from build123d import *

# Parameters (mm, degrees)
F0_R     = 3.5
F0_R_2   = 1.5
F1_DEPTH = 20
F2_W     = 5
F2_H     = 30
F3_DEPTH = 5


with BuildPart() as f1:
    # F0 (on Top) → F1 (new body)
    with BuildSketch(Plane.XY):
        Polygon((-10, 15), (-15, 15), (-15, -15), (-10, -15), (10, -15), (15, -15), (15, 15), (10, 15), align=None)
        with Locations((-5, -7.9105878249)):
            Circle(F0_R, mode=Mode.SUBTRACT)
        with Locations((5, -5.0300965086)):
            Circle(F0_R, mode=Mode.SUBTRACT)
        with Locations((-5, 0)):
            Circle(F0_R, mode=Mode.SUBTRACT)
        with Locations((-5, 7.8226719052)):
            Circle(F0_R, mode=Mode.SUBTRACT)
        with Locations((5, 4.2056075387)):
            Circle(F0_R, mode=Mode.SUBTRACT)
        with Locations((5, 4.2056075387)):
            Circle(F0_R)
        with Locations((5, 4.2056075387)):
            Circle(F0_R_2, mode=Mode.SUBTRACT)
        with Locations((-5, 7.8226719052)):
            Circle(F0_R)
        with Locations((-5, 7.8226719052)):
            Circle(F0_R_2, mode=Mode.SUBTRACT)
        with Locations((-5, 0)):
            Circle(F0_R)
        with Locations((-5, 0)):
            Circle(F0_R_2, mode=Mode.SUBTRACT)
        with Locations((-5, -7.9105878249)):
            Circle(F0_R)
        with Locations((-5, -7.9105878249)):
            Circle(F0_R_2, mode=Mode.SUBTRACT)
        with Locations((5, -5.0300965086)):
            Circle(F0_R)
        with Locations((5, -5.0300965086)):
            Circle(F0_R_2, mode=Mode.SUBTRACT)
    extrude(amount=F1_DEPTH)

    # F2 (on face) → F3 (join)
    with BuildSketch(Plane(origin=(0, 0, 0), x_dir=(1, 0, 0), z_dir=(0, 0, -1))):
        with Locations((12.5, 0)):
            Rectangle(F2_W, F2_H)
        with Locations((-12.5, 0)):
            Rectangle(F2_W, F2_H)
    extrude(amount=F3_DEPTH)


solid = f1.part
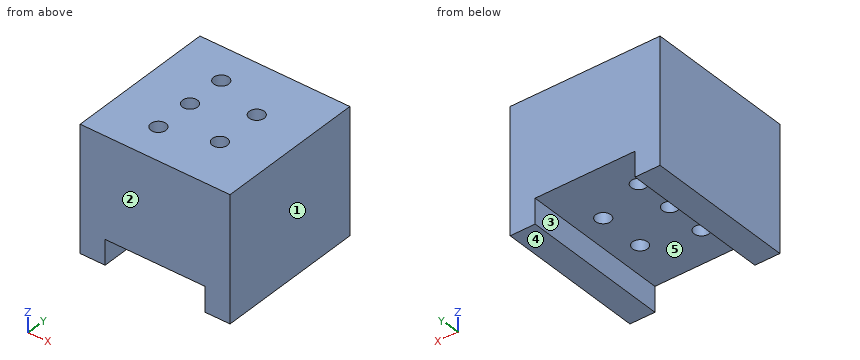
Part model, mm, in its own coordinate system. Face numbers are marked on the shaded views. A direction names the side the tool comes from. Coordinates: 2 decimals unless noted, no trailing zeros. Order: outer loops, then holes, each group sorted by start corner. A loop starts at its lowest first (then second) coordinate and runs counter-clockwise, first axis right, second up.
(1) Slice it at C-C, the plane y = 0. Write the cut outline in (x, z).
Check sheet entries:
outline: (-15, -5) - (-10, -5) - (-10, 0) - (-6.5, 0) - (-6.5, 20) - (-15, 20) - close; (-3.5, 0) - (10, 0) - (10, -5) - (15, -5) - (15, 20) - (-3.5, 20) - close
(2) Slice it at A-A, the plane x = 5. Write the cut outline in (y, z), and give its area (3 significant figures).
Check sheet entries:
outline: (-15, 0) - (-6.53, 0) - (-6.53, 20) - (-15, 20) - close; (-3.53, 0) - (2.71, 0) - (2.71, 20) - (-3.53, 20) - close; (5.71, 0) - (15, 0) - (15, 20) - (5.71, 20) - close
area: 480 mm2
(3) Pull direction X, two halves, no side cores. Call the marked faces 1, 2 and 3: pulls with the +X half, pulls with the -X half, needs draft (parallel to the pull), parting line crosses it, or undercut.
Check sheet entries:
face 1: pulls with the +X half
face 2: needs draft
face 3: undercut
(4) Slice it at D-D, the plane z = 8. Write the cut outline in (x, y), and give its area (3 significant figures).
Check sheet entries:
outline: (-15, -15) - (15, -15) - (15, 15) - (-15, 15) - close; hole circle Ø3 at (-5, -7.91); hole circle Ø3 at (-5, 0); hole circle Ø3 at (-5, 7.82); hole circle Ø3 at (5, -5.03); hole circle Ø3 at (5, 4.21)
area: 865 mm2
(5) Pin check, flat tips, straight feed: pin 1 Ø3.5 at (x, y) = (-5, 0) entering from -Z; pin 2 Ø2.5 at (x, y) = (-5, -7.91) entering from +Z. Stop position of each tip, or through.
Check sheet entries:
pin 1: stops at z = 0
pin 2: passes through
(6) Slice it at B-B, the plane x = -5. Write the cut outline in (y, z).
Check sheet entries:
outline: (-15, 0) - (-9.41, 0) - (-9.41, 20) - (-15, 20) - close; (-6.41, 0) - (-1.5, 0) - (-1.5, 20) - (-6.41, 20) - close; (1.5, 0) - (6.32, 0) - (6.32, 20) - (1.5, 20) - close; (9.32, 0) - (15, 0) - (15, 20) - (9.32, 20) - close
(7) Tool access for the marked faces 4 and 5: list every direction of +Z, -Z, +X, -X, +Y, -Y with a clear straight run to the whole face (end or side of a thin tool).
Check sheet entries:
face 4: -Z, +X, -X, +Y, -Y
face 5: -Z, +Y, -Y
(8) Probe L1, parallel to Y at x = -5, z = 10.75; L2, parallel to Y at x = 5, z = 12; L3, parallel to X at y = -8, z = 14.25. List the from-to ranges inside material, lowest first.
Check sheet entries:
L1: y = -15 to -9.41, -6.41 to -1.5, 1.5 to 6.32, 9.32 to 15
L2: y = -15 to -6.53, -3.53 to 2.71, 5.71 to 15
L3: x = -15 to -6.5, -3.5 to 15
